Answer from the drawing. Dimensions are ordinates in mm from the lowest x, y and z of the part. A direction names the side the tool comes from. Round coordinates to 2 decimals unless told otherwise and drop trailing zeros. Order: outer loops, then holes, each group sorted by start corner. A loop starts at its lowest first (then second) coordinate and runs counter-clockwise, first axis right, second up. Notation, with made-up numbers: M -3.5,-20 L 4.5,-20 A25 ccw 4.5,-2 Z; hole C 44,-31.75 d10. An arc over 180 degrees is marked long. Write item = value, one per line. Start each with the question number.
(1) Straight lines are drawn through the part: probe 1 along X at (y, z) = (1.7, 11); probe 2 along X at (y, z) = (22.5, 2); probe 3 along Y at (x, z) = (26, 1.15). For each, find the intervals that lie inside material, in ascending order. Write a range as from..to.
(2) A cutting plane is placed at A-A, the plane z = 16.5. Determine the outline of the cut face in (x, y).
(3) A cutting plane is placed at C-C, the plane z = 11. Determine the outline of the cut face in (x, y).
(4) Which of the six approach directions +Z, -Z, +X, -X, +Y, -Y give full straight-line access (tool end or side, diameter ignored) to the marked faces 1, 2, 3, 4 and 5?
(5) A cutting plane is placed at B-B, the plane y = 12.5. Determine the outline of the cut face in (x, z), and give its area (3 significant figures).
(6) A cutting plane is placed at D-D, the plane y = 3. Determine the outline of the cut face in (x, z).
(7) For a pull along Y with two mould halves and no side action, classify the marked faces 6, 7 and 8 as released by +Y, released by -Y, zero draft, split by the parting line, or undercut.
(8) Each of these flat-tipped pins is pushed along its axis until it touches: pin 1 (1 mm diameter, centred on x = 20, y = 17.5, fed in from +Z); pin 2 (6 mm diameter, centred on x = 27.5, z = 9.5, fed in from -Y); pin 3 (3 mm diameter, centred on y = 2.5, z = 5.5, fed in from -X). Where does it stop, or does it pass through?
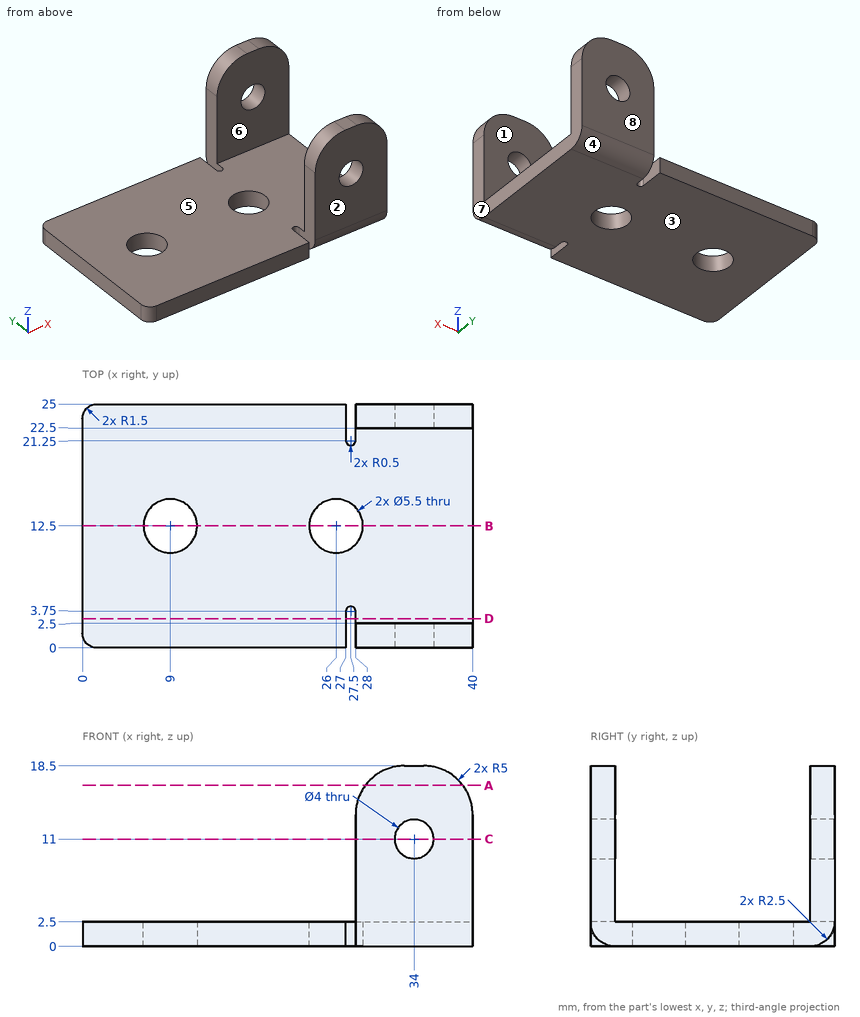
Reported:
q1.probe_1 = 28..32, 36..40
q1.probe_2 = 0..27, 28..40
q1.probe_3 = 0..9.75, 15.25..25
q2.outline = M 29,0 L 39,0 L 39,2.5 L 29,2.5 Z; M 29,22.5 L 39,22.5 L 39,25 L 29,25 Z
q3.outline = M 28,0 L 32,0 L 32,2.5 L 28,2.5 Z; M 28,22.5 L 32,22.5 L 32,25 L 28,25 Z; M 36,0 L 40,0 L 40,2.5 L 36,2.5 Z; M 36,22.5 L 40,22.5 L 40,25 L 36,25 Z
q4.face_1 = +Z, +X, -X
q4.face_2 = +Z, -Z, +X, -X, -Y
q4.face_3 = -Z, +X, -X, +Y, -Y
q4.face_4 = -Z, +X, +Y
q4.face_5 = +Z, -X
q5.outline = M 0,0 L 6.25,0 L 6.25,2.5 L 0,2.5 Z; M 11.75,0 L 23.25,0 L 23.25,2.5 L 11.75,2.5 Z; M 28.75,0 L 40,0 L 40,2.5 L 28.75,2.5 Z
q5.area = 72.5 mm²
q6.outline = M 0,0 L 27,0 L 27,2.5 L 0,2.5 Z; M 28,0 L 40,0 L 40,2.5 L 28,2.5 Z
q7.face_6 = undercut
q7.face_7 = zero draft
q7.face_8 = released by +Y
q8.pin_1 = 2.5
q8.pin_2 = 0
q8.pin_3 = 28
